The drawing under review shows one solid part. Ordinate dimensions are in mm from its lowest x, y, z. A direction names the side the tool comes from. Give positions to 0.01 mm unless a question says otherwise; leave off trailing zeros. Write each loop counter-clockwise with the first axis right and the second up, starting at its lowest first coordinate (ties: lowest second). Pieces come first, ordered by that corner, then holes.
Q1. We need section D-D (z = 46.5). Write out the cut boundary in (x, y), then the cut area to 3 significant figures.
Q2. We need section A-A (y = 21.25). Write out the cut boundary in (x, z).
Q3. For line 1 (Z direction, x = 7.5, y = 16.25); line 2 (X direction, y = 21.25, z = 75); line 3 (Y direction, x = 9, z = 37.5), list the stretches that pass through material, from the lowest coordinate up.
Q4. Mouldability with a two-part tool opening along X and no side actions: class the marked faces 3, 4, 5 and 6 as released by +X, released by -X, zero draft, split by the parting line, or undercut.
Q5. We need section C-C (x = 29). Write out the cut boundary in (y, z), then the cut area to 3 significant figures.
Q6. We need section B-B (z = 16.5). Write out the cut boundary in (x, y), then the cut area to 3 significant figures.
Q7. Insertion check: P1, Ø8, axis at x = 31, z = 39.5, coming from the +Y side; P2, Ø12, axis at x = 32.5, z = 71, coming from the +Y side; P3, Ø5, axis at x = 15.5, y = 17, coming from the -Z side. Each pin has a flat end and moves straight along its axis. Give the tip position at first contact, or say it passes through.
Q8. Machinability: for the marked faces 1 and 2, which of the approach directions +Z, -Z, +X, -X, +Y, -Y give a long, thin tool a straight path to every point of the face, cutting with its end or side? Answer none if there is none.
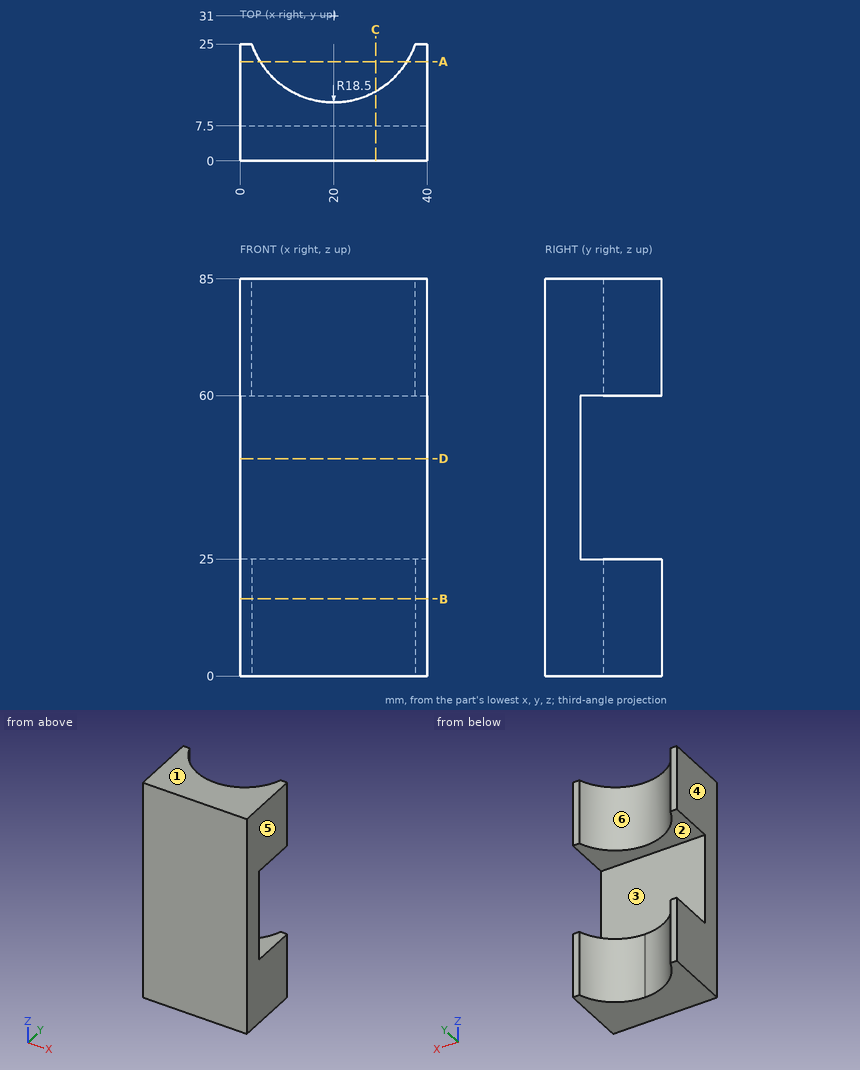
Computed:
1. outline: (0, 0) - (40, 0) - (40, 7.5) - (0, 7.5) - close
1. area: 300 mm2
2. outline: (0, 0) - (4.28, 0) - (4.28, 25) - (0, 25) - close; (0, 60) - (4.28, 60) - (4.28, 85) - (0, 85) - close; (35.72, 0) - (40, 0) - (40, 25) - (35.72, 25) - close; (35.72, 60) - (40, 60) - (40, 85) - (35.72, 85) - close
3. line 1: z = 0 to 25, 60 to 85
3. line 2: x = 0 to 4.28, 35.72 to 40
3. line 3: y = 0 to 7.5
4. face 3: zero draft
4. face 4: released by -X
4. face 5: released by +X
4. face 6: undercut
5. outline: (0, 0) - (14.84, 0) - (14.84, 25) - (7.5, 25) - (7.5, 60) - (14.84, 60) - (14.84, 85) - (0, 85) - close
5. area: 1,000 mm2
6. outline: (0, 0) - (40, 0) - (40, 25) - (37.5, 25) arc R18.5 cw to (2.5, 25) - (0, 25) - close
6. area: 680 mm2
7. P1: stops at y = 7.5
7. P2: stops at y = 25
7. P3: passes through
8. face 1: +Z, +X, -X, +Y, -Y
8. face 2: +X, -X, +Y
